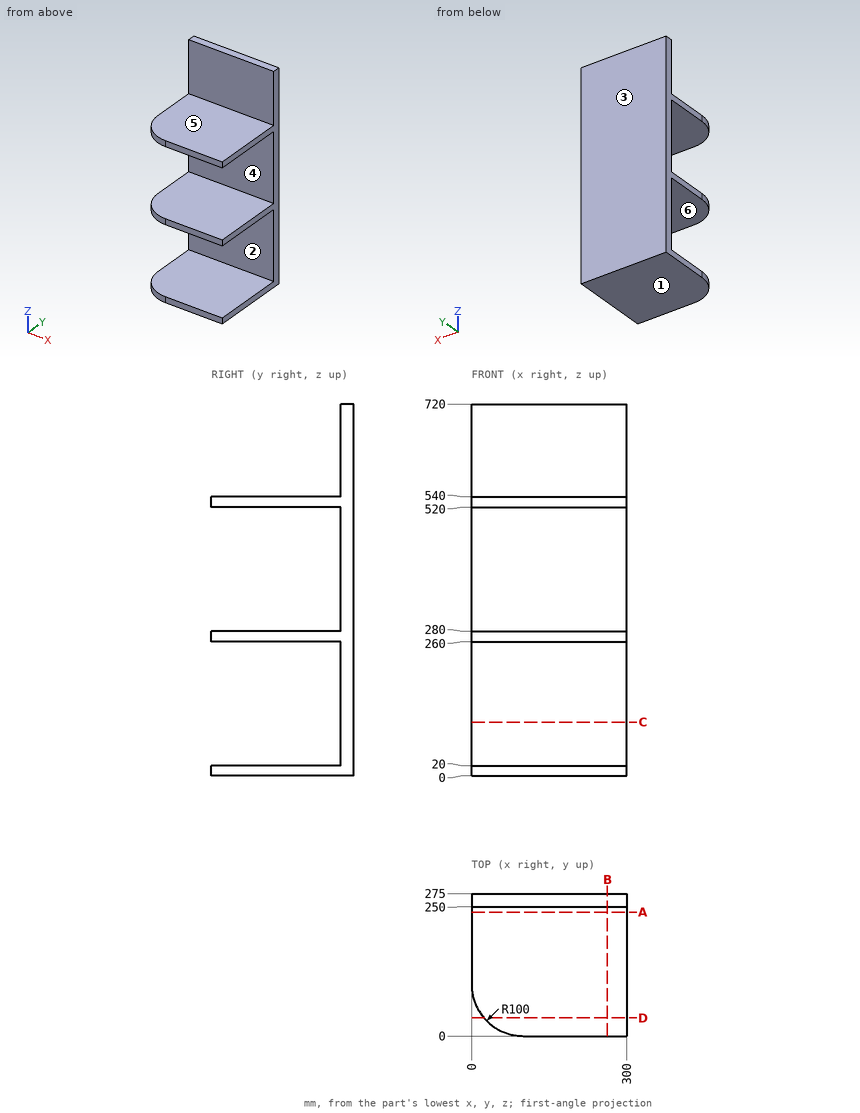
The drawing under review shows one solid part. Ordinate dimensions are in mm from its lowest x, y, z. A direction names the side the tool comes from. Round coordinates to 2 decimals unless told otherwise and drop trailing zeros. Order: outer loops, then holes, each group sorted by start corner. A loop starts at its lowest first (then second) coordinate and runs counter-clockwise, first axis right, second up. Notation, with made-up numbers: M 59,76 L 98,76 A15 cw 98,102 Z; hole C 27,63 d1. An arc over 180 degrees is marked long. Answer as CSV lines item,"result". Start each with the question number.
1) The part is to be moulded in two halves that separate along Z. For the marked faces 1, 2, 3 and 4, say which applies: +Z half, -Z half, draft (parallel to the pull), parting line (faces both ways), or undercut.
2) Add section C-C (z = 104). Give the boundary of the cut face in (x, y), then the cut area to 3 significant figures.
3) Add section A-A (y = 240). Give the boundary of the cut face in (x, z), then the cut area to 3 significant figures.
4) Wall thickness on line 1 along Z through (x, y) = (279.5, 67.5); line 2 along Y through (x, z) = (102, 541.5): over which ranges is each line inside the solid? List them lowest first. Write a range as [from, to].
5) Add section D-D (y = 35). Give the boundary of the cut face in (x, z).
6) For pin 1 Ø4 at (x, y) = (103.5, 239.5) entering from +Z, flat-tipped, find the tip position at first contact; note if it passes through.
7) Tool access review of the marked faces 5 and 6: name each direction out of +Z, -Z, +X, -X, +Y, -Y from which nothing blocks a thin tool from reaching the whole face with its end or side.
8) Add section B-B (x = 263). Give the boundary of the cut face in (y, z).
Resolved:
1,face 1,"-Z half"
1,face 2,"undercut"
1,face 3,"draft"
1,face 4,"undercut"
2,outline,"M 0,250 L 300,250 L 300,275 L 0,275 Z"
2,area,"7,500 mm^2"
3,outline,"M 0,0 L 300,0 L 300,20 L 0,20 Z; M 0,260 L 300,260 L 300,280 L 0,280 Z; M 0,520 L 300,520 L 300,540 L 0,540 Z"
3,area,"18,000 mm^2"
4,line 1,"[0, 20], [260, 280], [520, 540]"
4,line 2,"[250, 275]"
5,outline,"M 24.01,0 L 300,0 L 300,20 L 24.01,20 Z; M 24.01,260 L 300,260 L 300,280 L 24.01,280 Z; M 24.01,520 L 300,520 L 300,540 L 24.01,540 Z"
6,pin 1,"z = 540"
7,face 5,"+Z, +X, -X, -Y"
7,face 6,"+X, -X, -Y"
8,outline,"M 0,0 L 275,0 L 275,720 L 250,720 L 250,540 L 0,540 L 0,520 L 250,520 L 250,280 L 0,280 L 0,260 L 250,260 L 250,20 L 0,20 Z"
